Answer from the drawing. Dimensions are ordinates in mm from the lowest x, y and z of the part. A direction names the side the tool comes from. Give positions to 0.01 mm unless a question says otherwise; leave off trailing zeros. Order: outer loops, then holes, each group sorted by start corner. A loop starts at its lowest first (then second) coordinate and runs counter-clockwise, first axis right, second up.
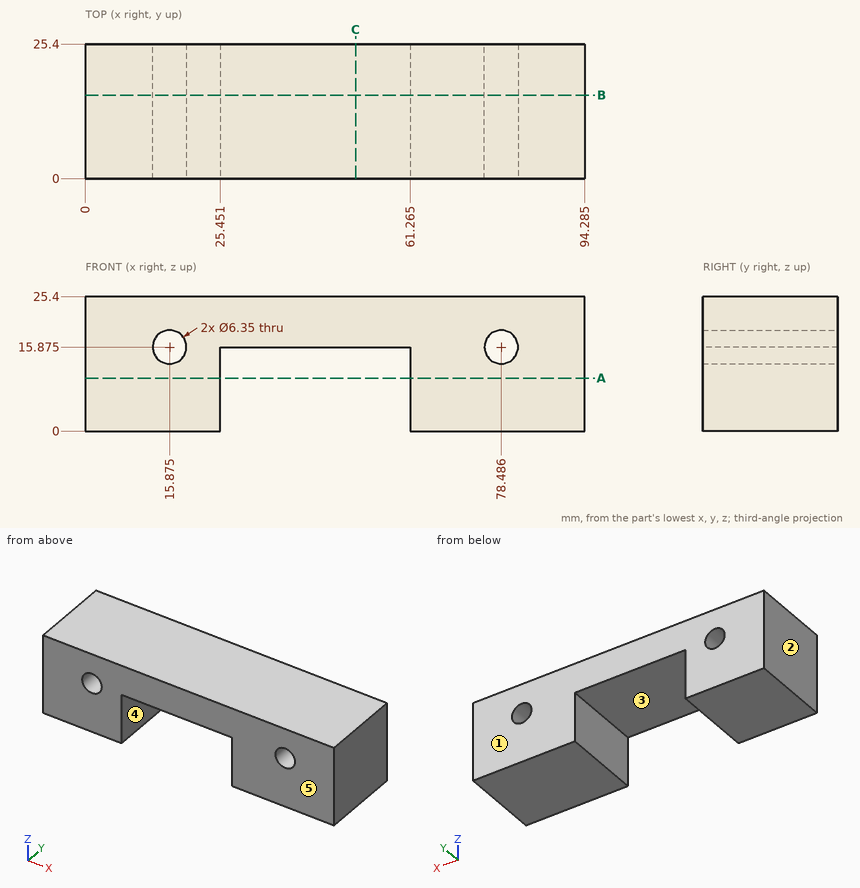
1. The part is cut by section C-C (x = 51). Write down the section's boundary in (y, z) (3 decimals).
Findings below:
outline: (0, 15.875) - (25.4, 15.875) - (25.4, 25.4) - (0, 25.4) - close
2. Which of the six approach directions +Z, -Z, +X, -X, +Y, -Y give full straight-line access (tool end or side, diameter ignored) to the marked faces 4 and 5?
Findings below:
face 4: -Z, +Y, -Y
face 5: +Z, -Z, +X, -X, -Y
3. The mould has two halves that part along X. Classify the marked faces 1, 2 and 3: pulls with the +X half, pulls with the -X half, needs draft (parallel to the pull), parting line crosses it, or undercut.
Findings below:
face 1: needs draft
face 2: pulls with the -X half
face 3: undercut
4. The part is cut by section A-A (z = 10). Write down the section's boundary in (x, y) (1 decimal).
Findings below:
outline: (0, 0) - (25.5, 0) - (25.5, 25.4) - (0, 25.4) - close; (61.3, 0) - (94.3, 0) - (94.3, 25.4) - (61.3, 25.4) - close
5. The part is cut by section B-B (y = 15.75). State how many separate pieces and enclosed holes the cut face has, then the cut area to 3 significant figures.
Findings below:
separate pieces: 1
enclosed holes: 2
area: 1,760 mm2
6. Straight lines are drawn through the part: probe 1 along X at (y, z) = (21.25, 10.5) (1 decimal); probe 2 along X at (y, z) = (9.75, 17) (1 decimal); probe 3 along Z at (x, y) = (32, 11.5) (3 decimals). For each, find the intervals that lie inside material, in ascending order.
Findings below:
probe 1: x = 0 to 25.5, 61.3 to 94.3
probe 2: x = 0 to 12.9, 18.8 to 75.5, 81.5 to 94.3
probe 3: z = 15.875 to 25.4
